from build123d import *

# Parameters (mm, degrees)
CUT_EXTRUDE1_DEPTH = 1
FILLET1_R          = 1.5
CHAMFER1_SIZE      = 0.5


with BuildPart() as part:
    # Sketch1 → Revolve1 (revolve)
    with BuildSketch(Plane(origin=(0, 0, 0), x_dir=(1, 0, 0), z_dir=(0, 1, 0))):
        Polygon((0, 0), (-6, -7.3e-16), (-6, -1.5000000000000007), (1e-17, -1.5), align=None)
        Polygon((1e-17, 1.3999999999999995), (1e-17, 0), (1e-17, -1.5), (2, -1.5), (2, 1.3999999999999995), align=None)
    revolve(axis=Axis((1e-17, 0, 1.5), (-1, 0, 1.1e-16)))

    # Sketch3 → Cut-Extrude1 (cut)
    with BuildSketch(Plane(origin=(2, 0, -2.2e-16), x_dir=(-1.3e-16, 0, -1), z_dir=(1, 0, -1.3e-16))):
        Polygon((-2.2216878364870323, -1.2500000000000002), (-0.7783121635129678, -1.2500000000000002), (-0.05662432702593554, 0), (-0.7783121635129678, 1.2500000000000002), (-2.2216878364870323, 1.2500000000000004), (-2.9433756729740645, 0), align=None)
    extrude(amount=-CUT_EXTRUDE1_DEPTH, mode=Mode.SUBTRACT)

    # Fillet1
    fillet1_edges = [part.edges().sort_by_distance(p)[0] for p in [
        (2.000000000000001, -3.6e-16, 4.3999999999999995),
    ]]
    fillet(fillet1_edges, radius=FILLET1_R - 0.0001)  # a hair under: the kernel refuses the full size

    # Chamfer1
    chamfer1_edges = [part.edges().sort_by_distance(p)[0] for p in [
        (-6, -1.8e-16, 3.000000000000001),
    ]]
    chamfer(chamfer1_edges, length=CHAMFER1_SIZE)


solid = part.part
The listing builds one solid part. Answer for the finished solid, in the listing's coordinates (mm). A direction names the side the tool comes from. Give positions to 0.01 mm unless a question says otherwise; leave off trailing zeros. Write each loop counter-clockwise with the first axis right and the second up, starting at its lowest first coordinate (ties: lowest second). Pieces come first, ordered by that corner, then holes.
1) For a pull along Y with two mould halves and no side action, classify faces 3 (the face through (0.2, -2, 3.6)), 4 (the face through (1.5, -1.25, 1.5)), 5 (the face through (-6, 0, 2)) as pulls with the +Y half, pulls with the -Y half, needs draft (parallel to the pull), parting line crosses it, or undercut.
2) Find the intervals of material crossed by L1, parallel to Z at x = -2, y = 0.4; L2, parallel to Z at x = 1.5, y = 1.2; L3, parallel to X at y = 0.25, z = 2.5, in increasing order.
3) Section B-B (x = 0.25) is taken. Write down the section's boundary in (y, z).
4) Given P1, Ø1.5, axis at x = -2.5, z = 1, coming from the +Y side; P2, Ø2, axis at x = -5, y = 1, coming from the +Z side; P3, Ø1.5, axis at y = 2, z = 1, coming from the -X side, each flat-ended and moving along its own axis, determine where each tip first touches the part or whether it passes through.
5) Section A-A (x = -3) is taken. Write down the section's boundary in (y, z).
6) A tool of negligible diameter and unlimited length cuts with its end or side. For faces 1 (the face through (1, 0, 2)), 2 (the face through (0, 1, 0)), from which of +Z, -Z, +X, -X, +Y, -Y can it reach the whole face along a straight path? Write none if from no direction.
Response:
1. face 3: parting line crosses it
1. face 4: undercut
1. face 5: needs draft
2. L1: z = 0.05 to 2.95
2. L2: z = -0.71 to 0.75, 2.25 to 3.71
2. L3: x = -5.97 to 1
3. outline: circle Ø5.8 at (0, 1.5)
4. P1: stops at y = 1.5
4. P2: stops at z = 3
4. P3: stops at x = -5.69
5. outline: circle Ø3 at (0, 1.5)
6. face 1: +X
6. face 2: -X
